from build123d import *

# Parameters (mm, degrees)
BOSS_EXTRUDE1_DEPTH                               = 150
CSK_FOR_4_FLAT_HEAD_MACHINE_SCREW_100_D           = 3.2639
CSK_FOR_4_FLAT_HEAD_MACHINE_SCREW_100_CSINK_D     = 5.715
CSK_FOR_4_FLAT_HEAD_MACHINE_SCREW_100_CSINK_ANGLE = 100
CSK_FOR_4_FLAT_HEAD_MACHINE_SCREW_2_D             = 3.2639
CSK_FOR_4_FLAT_HEAD_MACHINE_SCREW_2_CSINK_D       = 5.715
CSK_FOR_4_FLAT_HEAD_MACHINE_SCREW_2_CSINK_ANGLE   = 100
FILLET1_R                                         = 1
F_2_CLEARANCE_HOLE1_AT_2_COUNT                    = 2
F_2_CLEARANCE_HOLE1_AT_2_PITCH                    = 4.8


with BuildPart() as part:
    # Sketch2 → Boss-Extrude1 (new, symmetric)
    with BuildSketch(Plane.XY):
        with BuildLine():
            Line((-9.525, 0), (9.525, 0))
            Line((9.525, 0), (9.525, 19.05))
            Line((9.525, 19.05), (8.73125, 19.05))
            ThreePointArc((8.73125, 19.05), (8.169983992, 18.817516008), (7.9375, 18.25625))
            Line((7.9375, 18.25625), (7.9375, 2.38125))
            ThreePointArc((7.9375, 2.38125), (7.705016008, 1.819983992), (7.14375, 1.5875))
            Line((7.14375, 1.5875), (-8.73125, 1.5875))
            ThreePointArc((-8.73125, 1.5875), (-9.292516008, 1.355016008), (-9.525, 0.79375))
            Line((-9.525, 0.79375), (-9.525, 0))
        make_face()
    extrude(amount=BOSS_EXTRUDE1_DEPTH, both=True)

    # CSK for _4 Flat Head Machine Screw _100 (through all)
    with Locations(Plane(origin=(0, 0, 0), x_dir=(-1, 0, 0), z_dir=(0, -1, 0))):
        with Locations((4.0625, -146), (4.0625, 146)):
            CounterSinkHole(CSK_FOR_4_FLAT_HEAD_MACHINE_SCREW_100_D / 2, CSK_FOR_4_FLAT_HEAD_MACHINE_SCREW_100_CSINK_D / 2, counter_sink_angle=CSK_FOR_4_FLAT_HEAD_MACHINE_SCREW_100_CSINK_ANGLE)

    # CSK for _4 Flat Head Machine Screw _ 2 (through all)
    with Locations(Plane(origin=(9.525, 0, 0), x_dir=(0, 0, -1), z_dir=(1, 0, 0))):
        with Locations((-146, 13.5875), (146, 13.5875)):
            CounterSinkHole(CSK_FOR_4_FLAT_HEAD_MACHINE_SCREW_2_D / 2, CSK_FOR_4_FLAT_HEAD_MACHINE_SCREW_2_CSINK_D / 2, counter_sink_angle=CSK_FOR_4_FLAT_HEAD_MACHINE_SCREW_2_CSINK_ANGLE)

    # Fillet1
    fillet1_edges = [part.edges().sort_by_distance(p)[0] for p in [
        (9.525, 0, 0),
    ]]
    fillet(fillet1_edges, radius=FILLET1_R)

    # Sketch30 → #2 Clearance Hole1 (revolve, cut)
    with BuildSketch(Plane(origin=(3.49375, 1.5875, 129.88), x_dir=(0, 0, 1), z_dir=(1, 0, 0))):
        Polygon((0, 0), (0, 1.5875), (2.0574, 1.5875), (1.2192, 0.623261201), (1.2192, 0), align=None)
    f_2_clearance_hole1 = revolve(axis=Axis((3.49375, 7.9375, 129.88), (0, -1, 0)), mode=Mode.SUBTRACT)

    # #2 Clearance Hole1 at 2: #2 Clearance Hole1 ×2
    with Locations(*[(0, 0, -i * F_2_CLEARANCE_HOLE1_AT_2_PITCH) for i in range(1, F_2_CLEARANCE_HOLE1_AT_2_COUNT)]):
        add(f_2_clearance_hole1, mode=Mode.SUBTRACT)


solid = part.part
Design review of the part built by this model. Coordinates are the model's own, in mm. A direction names the side the tool comes from. Round coordinates to 2 decimals unless told otherwise and drop trailing zeros. Write each loop counter-clockwise with the first axis right and the second up, starting at its lowest first coordinate (ties: lowest second). Pieces come first, ordered by that corner, then holes.
Item 1: Wall thickness on L1, parallel to Z at x = -4.25, y = 1; L2, parallel to Y at x = 4.25, z = -62; L3, parallel to X at y = 1.4, z = 129.88 (3 decimals): over which ranges is each line inside the solid? List them lowest first.
Item 2: For pin 1 Ø3 at (x, z) = (-4.06, -146) entering from +Y; pin 2 Ø2 at (y, z) = (17, 90.5) entering from -X; pin 3 Ø3 at (x, z) = (3.49, 125.08) entering from -Y; pin 4 Ø4 at (y, z) = (13.59, -146) entering from +X, all flat-tipped, find the tip position at first contact; note any pin that passes through.
Item 3: Consider section B-B on y = 6.25. Give the boundary of the cut face in (x, z) (1 decimal).
Item 4: For faces 1 (the flat face through (7.938, 10, 2)), 2 (the flat face through (-1, 0, 2)), list the 3-axis set-ups (+Z, -Z, +X, -X, +Y, -Y) from which the entire face can be reached by the end or side of a thin tool; tool diameter is ignored.
Check values:
1. L1: z = -150 to -147.66, -144.34 to 144.34, 147.66 to 150
1. L2: y = 0 to 1.59
1. L3: x = -9.244 to 2.275, 4.713 to 9.525
2. pin 1: passes through
2. pin 2: stops at x = 7.94
2. pin 3: stops at y = 0.64
2. pin 4: stops at x = 8.81
3. outline: (7.9, -150) - (9.5, -150) - (9.5, 150) - (7.9, 150) - close
4. face 1: +Z, -Z, -X, +Y
4. face 2: +Z, -Z, +X, -X, -Y
